Read the model definition and answer for the solid it produces. Units are mm, in the model's axes. A direction names the side the tool comes from. Give positions to 0.01 mm unless a question says otherwise; leave off trailing zeros. Write each loop counter-clockwise with the first axis right and the second up, starting at its lowest first coordinate (ties: lowest second). Pieces come first, ordered by that corner, then holes. Notation, with made-up numbers: (-9, 30) -> (10, 30) arc R22 ccw to (10, 64) -> close; hole circle Ø2 at (0, 45.25). An arc over 180 degrees is marked (long way). Answer as CSV lines item,"result". Start each with the question number.
1. The part is cut by section A-A, the plane y = 2.25. Determine the outline of the cut face in (x, z), and give its area (3 significant figures).
2. The part is cut by section C-C, the plane z = -2.5. Determine the outline of the cut face in (x, y).
3. For a pull along Z with two mould halves and no side action, classify faces 4 (the flat face through (5.25, 6, -12)), 5 (the flat face through (0, 1, 17)), 6 (the cylindrical face through (10.12, 0.74, -12.59)) as pulls with the +Z half, pulls with the -Z half, needs draft (parallel to the pull), parting line crosses it, or undercut.
4. The part is cut by section D-D, the plane x = 0.75. Determine the outline of the cut face in (y, z), and give its area (3 significant figures).
5. Find the intervals of material crossed by line 1 (Z direction, x = -0.25, y = 9.75); line 2 (X direction, y = 1, z = -14.25); line 3 (Z direction, x = 9.75, y = 0.8), in increasing order.
6. The part is cut by section B-B, the plane x = 10.75. Determine the outline of the cut face in (y, z), and give its area (3 significant figures).
7. A tool of negligible diameter and unlimited length cuts with its end or side. For faces 1 (the flat face through (0, 6, 4.5)), 2 (the flat face through (12, 11, -2)), 3 (the flat face through (0, 6, 12.5)), from which of +Z, -Z, +X, -X, +Y, -Y can it reach the whole face along a straight path? Write none if from no direction.
8. Given pin 1 (6 mm diameter, centred on x = -2, z = 0.5, fed in from -Y); pin 2 (8 mm diameter, centred on x = 7, y = 16, fed in from -Z); pin 3 (5 mm diameter, centred on x = 0.5, y = 7.5, fed in from -Z); pin 4 (6.5 mm diameter, centred on y = 7.5, z = 8, fed in from -X), each flat-ended and moving along its own axis, determine where each tip first touches the part or whether it passes through.
from build123d import *

# Parameters (mm, degrees)
SKIZZE2_W                       = 25
SKIZZE2_H                       = 34
AUFSATZ_LINEAR_AUSTRAGEN1_DEPTH = 1.5
VERRUNDUNG1_R                   = 3
DURCHGANGSLOCH_F_R_M31_D        = 3.4
SKIZZE5_W                       = 24
SKIZZE5_H                       = 5
AUFSATZ_LINEAR_AUSTRAGEN2_DEPTH = 20
SKIZZE6_W                       = 10.5
SKIZZE6_H                       = 8
SKIZZE6_W_2                     = 15.3
AUFSATZ_LINEAR_AUSTRAGEN3_DEPTH = 10


with BuildPart() as part:
    # Skizze2 → Aufsatz-Linear austragen1 (new body)
    with BuildSketch(Plane(origin=(0, 0, 0), x_dir=(1, 0, 0), z_dir=(0, 1, 0))):
        Rectangle(SKIZZE2_W, SKIZZE2_H)
    extrude(amount=AUFSATZ_LINEAR_AUSTRAGEN1_DEPTH)

    # Verrundung1
    verrundung1_edges = [part.edges().sort_by_distance(p)[0] for p in [
        (12.5, 0.75, 17),
        (-12.5, 0.75, 17),
        (-12.5, 0.75, -17),
        (12.5, 0.75, -17),
    ]]
    fillet(verrundung1_edges, radius=VERRUNDUNG1_R)

    # Durchgangsloch für M31 (through all)
    with Locations(Plane(origin=(0, 1.5, 0), x_dir=(1, 0, 0), z_dir=(0, 1, 0))):
        with Locations((-9.75, 14.25), (9.75, 14.25), (9.75, -14.25), (-9.75, -14.25)):
            Hole(DURCHGANGSLOCH_F_R_M31_D / 2)

    # Skizze5 → Aufsatz-Linear austragen2 (add)
    with BuildSketch(Plane(origin=(0, 1.5, 0), x_dir=(1, 0, 0), z_dir=(0, 1, 0))):
        with Locations((0, 2.5)):
            Rectangle(SKIZZE5_W, SKIZZE5_H)
    extrude(amount=AUFSATZ_LINEAR_AUSTRAGEN2_DEPTH)

    # Skizze6 → Aufsatz-Linear austragen3 (add)
    with BuildSketch(Plane(origin=(0, 1.5, 0), x_dir=(1, 0, 0), z_dir=(0, 1, 0))):
        with Locations((0, 12.4)):
            Rectangle(SKIZZE6_W, SKIZZE6_H)
        with Locations((0, -8.5)):
            Rectangle(SKIZZE6_W_2, SKIZZE6_H)
    extrude(amount=AUFSATZ_LINEAR_AUSTRAGEN3_DEPTH)


solid = part.part
Results found:
1,outline,"(-12, -5) -> (12, -5) -> (12, 0) -> (-12, 0) -> close; (-7.65, 4.5) -> (7.65, 4.5) -> (7.65, 12.5) -> (-7.65, 12.5) -> close; (-5.25, -16.4) -> (5.25, -16.4) -> (5.25, -8.4) -> (-5.25, -8.4) -> close"
1,area,"326 mm²"
2,outline,"(-12.5, 0) -> (12.5, 0) -> (12.5, 1.5) -> (12, 1.5) -> (12, 21.5) -> (-12, 21.5) -> (-12, 1.5) -> (-12.5, 1.5) -> close"
3,face 4,"needs draft"
3,face 5,"pulls with the +Z half"
3,face 6,"undercut"
4,outline,"(0, -17) -> (1.5, -17) -> (1.5, -16.4) -> (11.5, -16.4) -> (11.5, -8.4) -> (1.5, -8.4) -> (1.5, -5) -> (21.5, -5) -> (21.5, 0) -> (1.5, 0) -> (1.5, 4.5) -> (11.5, 4.5) -> (11.5, 12.5) -> (1.5, 12.5) -> (1.5, 17) -> (0, 17) -> close"
4,area,"311 mm²"
5,line 1,"z = -16.4 to -8.4, -5 to 0, 4.5 to 12.5"
5,line 2,"x = -12.49 to -11.45, -8.05 to 8.05, 11.45 to 12.49"
5,line 3,"z = -16.99 to -15.95, -12.55 to 12.55, 15.95 to 16.99"
6,outline,"(0, -16.73) -> (1.5, -16.73) -> (1.5, -15.62) -> (0, -15.62) -> close; (0, -12.88) -> (1.5, -12.88) -> (1.5, -5) -> (21.5, -5) -> (21.5, 0) -> (1.5, 0) -> (1.5, 12.88) -> (0, 12.88) -> close; (0, 15.62) -> (1.5, 15.62) -> (1.5, 16.73) -> (0, 16.73) -> close"
6,area,"142 mm²"
7,face 1,"+X, -X, +Y"
7,face 2,"+Z, -Z, +X, +Y"
7,face 3,"+Z, +X, -X, +Y"
8,pin 1,"stops at y = 0"
8,pin 2,"stops at z = -5"
8,pin 3,"stops at z = -16.4"
8,pin 4,"stops at x = -7.65"
